```python
from build123d import *

# Parameters (mm, degrees)
SALIENTE_EXTRUIR1_DEPTH      = 2
SALIENTE_EXTRUIR1_DEPTH_BACK = 2
CROQUIS1_R                   = 7.5
CORTAR_EXTRUIR1_DEPTH        = 2.5
MATRIZC1_COUNT               = 48
CROQUIS3_R                   = 9
SALIENTE_EXTRUIR2_DEPTH      = 1
SALIENTE_EXTRUIR3_START      = 1
CROQUIS4_R                   = 9
SALIENTE_EXTRUIR3_DEPTH      = 1
CROQUIS5_R                   = 2.5
SALIENTE_EXTRUIR4_DEPTH      = 5
SALIENTE_EXTRUIR5_START      = 5
CROQUIS6_R                   = 2.5
SALIENTE_EXTRUIR5_DEPTH      = 5


with BuildPart() as part:
    # Croquis1 → Saliente-Extruir1 (new, two sides: drawn at the far end of the back side and taken through both)
    with BuildSketch(Plane.XY.offset(-SALIENTE_EXTRUIR1_DEPTH_BACK)):
        Circle(CROQUIS1_R)
    extrude(amount=SALIENTE_EXTRUIR1_DEPTH + SALIENTE_EXTRUIR1_DEPTH_BACK)

    # Croquis2 → Cortar-Extruir1 (cut, symmetric)
    with BuildSketch(Plane.XY):
        Polygon((-0.5, 7.5), (0.5, 7.5), (0, 6.633974596), align=None)
    cortar_extruir1 = extrude(amount=CORTAR_EXTRUIR1_DEPTH, both=True, mode=Mode.SUBTRACT)

    # MatrizC1: Cortar-Extruir1 ×48 about axis
    matrizc1_axis = Axis((0, 0, 0), (0, 0, 1))
    for i in range(1, MATRIZC1_COUNT):
        add(cortar_extruir1.rotate(matrizc1_axis, i * 360 / MATRIZC1_COUNT), mode=Mode.SUBTRACT)

    # Croquis3 → Saliente-Extruir2 (add)
    with BuildSketch(Plane.XY.offset(2)):
        Circle(CROQUIS3_R)
    extrude(amount=SALIENTE_EXTRUIR2_DEPTH)

    # Croquis4 → Saliente-Extruir3 (add)
    with BuildSketch(Plane(origin=(0, 0, -2), x_dir=(-1, 0, 0), z_dir=(0, 0, -1)).offset(SALIENTE_EXTRUIR3_START)):
        with Locations(Location((0, 0, 0), (0, 0, 180))):
            Circle(CROQUIS4_R)
    extrude(amount=-SALIENTE_EXTRUIR3_DEPTH)

    # Croquis5 → Saliente-Extruir4 (add)
    with BuildSketch(Plane.XY.offset(3)):
        Circle(CROQUIS5_R)
    extrude(amount=SALIENTE_EXTRUIR4_DEPTH)

    # Croquis6 → Saliente-Extruir5 (add)
    with BuildSketch(Plane(origin=(0, 0, -3), x_dir=(-1, 0, 0), z_dir=(0, 0, -1)).offset(SALIENTE_EXTRUIR5_START)):
        with Locations(Location((0, 0, 0), (0, 0, 180))):
            Circle(CROQUIS6_R)
    extrude(amount=-SALIENTE_EXTRUIR5_DEPTH)


solid = part.part
```
Model file for the job. Use its own axes, mm. Coordinates: 2 decimals unless noted, no trailing zeros. Order: outer loops, then holes, each group sorted by start corner. A loop starts at its lowest first (then second) coordinate and runs counter-clockwise, first axis right, second up. Notation, with made-up numbers: M 4.25,45.25 L 57.25,45.25 A33 cw 57.25,79.25 Z; hole C -28,27 d4. An arc over 180 degrees is marked long. Answer as CSV lines item,"result".
(1) Band-saw the part on C-C, the plane x = -2. List the corners of the cut face in (y, z).
Geometry says:
outline,"M -8.77,-3 L -1.5,-3 L -1.5,-8 L 1.5,-8 L 1.5,-3 L 8.77,-3 L 8.77,-2 L 6.69,-2 L 6.69,2 L 8.77,2 L 8.77,3 L 1.5,3 L 1.5,8 L -1.5,8 L -1.5,3 L -8.77,3 L -8.77,2 L -6.69,2 L -6.69,-2 L -8.77,-2 Z"
(2) Pull direction X, two halves, no side cores. Call faces 1 (the flat face through (2, 2, -3)), 2 (the flat face through (3.74, -5.99, 0.03)), 3 (the cylindrical face through (-1.172, 8.923, 2.493)): +X half, -X half, draft (parallel to the pull), parting line (faces both ways), or undercut.
Geometry says:
face 1,"draft"
face 2,"undercut"
face 3,"parting line"
(3) Band-saw the part on D-D, the plane z = 2.25. List the corners of the cut face in (x, y), then the cut area to 3 significant figures.
Geometry says:
outline,"C 0,0 d18"
area,"254 mm2"
(4) Band-saw the part on B-B, the plane z = -3.75. List the corners of the cut face in (x, y).
Geometry says:
outline,"C 0,0 d5"
(5) Flat gauge pins, fed straight in: pin 1 (1.1 mm diameter, centred on y = 6.5, z = 0.5, fed in from -X); pin 2 (1.1 mm diameter, centred on y = -6, z = 0, fed in from -X); pin 3 (0.5 mm diameter, centred on x = -6, z = 0, fed in from +Y). Where does each tip first touch, or does it go through?
Geometry says:
pin 1,"stops at x = -4.17"
pin 2,"stops at x = -4.94"
pin 3,"stops at y = 4.17"
(6) Wall check: line 1 along Z through (x, y) = (-6.5, -3.5); line 2 along Z through (x, y) = (-5.25, 3); line 3 along X through (y, z) = (-2.25, 4.5). Give the ranges that are in metal, low to high.
Geometry says:
line 1,"z = -3 to -2, 2 to 3"
line 2,"z = -3 to 3"
line 3,"x = -1.09 to 1.09"
(7) Band-saw the part on A-A, the plane y = 7.75. List the corners of the cut face in (x, z), then the cut area to 3 significant figures.
Geometry says:
outline,"M -4.58,-3 L 4.58,-3 L 4.58,-2 L -4.58,-2 Z; M -4.58,2 L 4.58,2 L 4.58,3 L -4.58,3 Z"
area,"18.3 mm2"
